Model file for the job. Use its own axes, mm. A direction names the side the tool comes from. Round coordinates to 2 decimals unless told otherwise and drop trailing zeros. Loops run counter-clockwise (first coordinate to the right, second up) from the corner with the lowest first, then second, coordinate; pieces in that order, holes last. Notation, with made-up numbers: (-24.75, -24) - (-8.75, -24) arc R26 cw to (-8.75, -4) - close; hole circle Ø6 at (82.5, 77.5). An arc over 180 degrees is marked (long way). Answer as a JSON object with one key per item and string values.
from build123d import *

# Parameters (mm, degrees)
F0_R      = 8.547489
F1_DEPTH  = 76.2
F1_FACE_W = 76.2
F1_FACE_H = 74.485234
F2_DEPTH  = 99.161685


with BuildPart() as f1:
    # F0 (on Front) → F1 (new body)
    with BuildSketch(Plane.XZ):
        with BuildLine():
            Line((-19.700978, 37.242617), (-19.842371, 37.242617))
            Line((-19.842371, 37.242617), (-19.842371, -37.242617))
            Line((-19.842371, -37.242617), (19.842371, -37.242617))
            Line((19.842371, -37.242617), (19.842371, 37.242617))
            Line((19.842371, 37.242617), (19.700978, 37.242617))
            ThreePointArc((19.700978, 37.242617), (0, 56.943595), (-19.700978, 37.242617))
        make_face()
        with Locations((0, 37.242617)):
            Circle(F0_R, mode=Mode.SUBTRACT)
        with Locations((0, 37.242617)):
            Circle(F0_R)
    extrude(amount=F1_DEPTH)

    # F1_face (on face) → F2 (join)
    with BuildSketch(Plane(origin=(-19.842371, -38.1, 0), x_dir=(0, -1, 0), z_dir=(-1, 0, 0))):
        Rectangle(F1_FACE_W, F1_FACE_H)
    extrude(amount=F2_DEPTH)


solid = f1.part
1) Slice it at A-A on y = -34.5. List the corners of the cut face in (x, z).
Values follow:
{"outline": "(-119, -37.24) - (19.84, -37.24) - (19.84, 37.24) - (19.7, 37.24) arc R19.7 ccw to (-19.7, 37.24) - (-119, 37.24) - close"}
2) Drop flat-ended pins along their axis: P1, Ø4, axis at x = 2, y = -27, coming from the +Z side; P2, Ø5, axis at y = -68, z = 46.5, coming from the -X side. Give the stop position or say it passes through.
Values follow:
{"P1": "z = 56.94", "P2": "x = -18.51"}
3) Tool access for faces 1 (the flat face through (-49, -38, -37.243)), 2 (the flat face through (-69, -38, 37.243)): list every direction of +Z, -Z, +X, -X, +Y, -Y with a clear straight run to the whole face (end or side of a thin tool).
Values follow:
{"face 1": "-Z, +X, -X, +Y, -Y", "face 2": "+Z, -X, +Y, -Y"}
4) Slice it at C-C on z = 45.5. List the corners of the cut face in (x, y).
Values follow:
{"outline": "(-17.89, -76.2) - (17.89, -76.2) - (17.89, 0) - (-17.89, 0) - close"}
5) Slice it at B-B on x = -42. List the corners of the cut face in (y, z), then the cut area to 3 significant figures.
Values follow:
{"outline": "(-76.2, -37.24) - (0, -37.24) - (0, 37.24) - (-76.2, 37.24) - close", "area": "5,680 mm²"}
6) Probe probe 1 along Z at (x, y) = (-59, -7); probe 2 along X at (y, z) = (-42, 41.5); probe 3 along Z at (x, y) = (7.5, -64). List the from-to ranges inside material, lowest first.
Values follow:
{"probe 1": "-37.24 to 37.24", "probe 2": "-19.24 to 19.24", "probe 3": "-37.24 to 55.46"}
